Verification items for this drawing (mm, ordinates from the low corner). A direction names the side the tool comes from. Round coordinates to 2 decimals unless told otherwise and drop trailing zeros. Write each loop counter-clockwise with the first axis right and the second up, starting at its lowest first coordinate (ties: lowest second). Pieces come first, ordered by that corner, then holes. Notation, with made-up numbers: M 33,62 L 56,62 A18 ccw 56,85 Z; hole C 80,-14 d7. An arc over 180 degrees is marked long. Write each question's results on one line, items separated by ' | '.
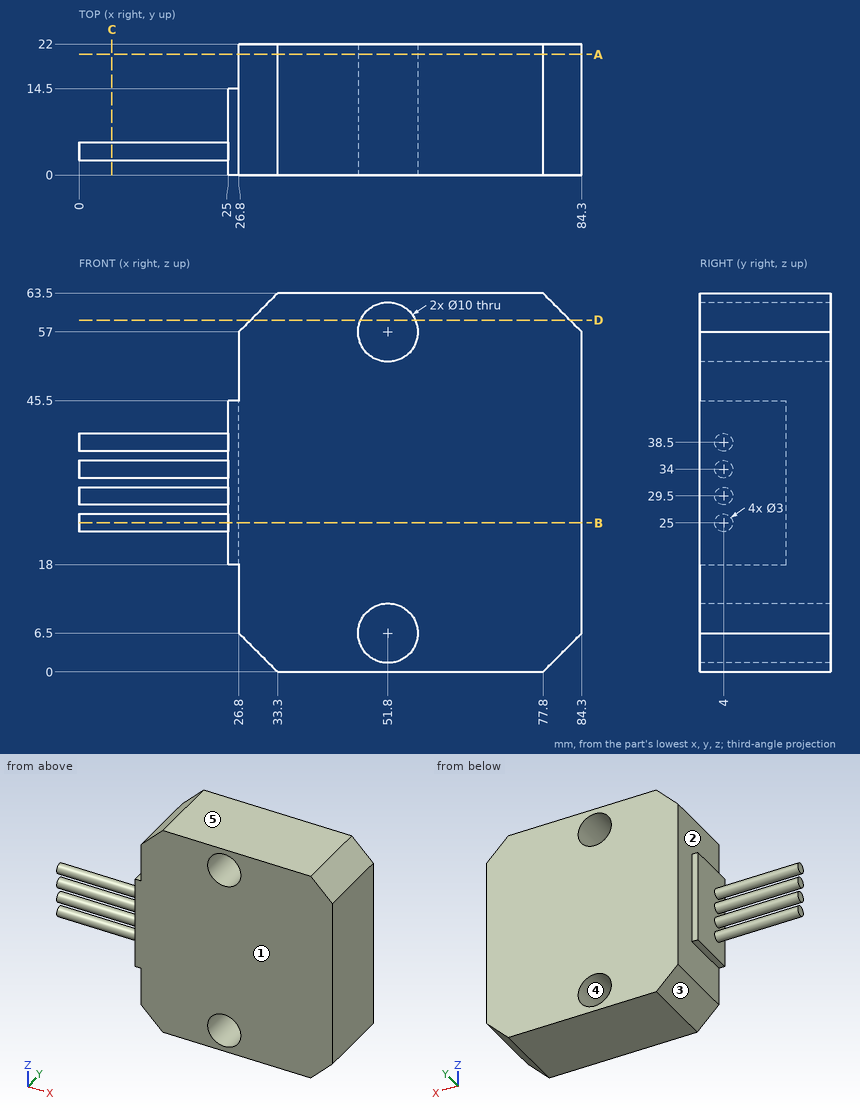
1) Material ranges on line 1 (X direction, y = 16.5, z = 6.5); line 2 (Z direction, x = 55, y = 16.75); line 3 (Z direction, x = 53, y = 4), recorded low to high. Write a range as [from, to].
Calculated:
line 1: x = [26.8, 46.8], [56.8, 84.3] | line 2: z = [0, 2.66], [10.34, 53.16], [60.84, 63.5] | line 3: z = [0, 1.65], [11.35, 52.15], [61.85, 63.5]
2) Access from +Z, -Z, +X, -X, +Y, -Y to the whole of each face (thin tool, end or side, straight path). Record for the marked faces 1 and 2.
Calculated:
face 1: +Z, -Z, +X, -X, -Y | face 2: -X, +Y
3) Sectioned sample at D-D, the plane z = 59. Record the cut outline in (x, y), and give its area (3 significant figures).
Calculated:
outline: M 28.8,0 L 47.22,0 L 47.22,22 L 28.8,22 Z; M 56.38,0 L 82.3,0 L 82.3,22 L 56.38,22 Z | area: 975 mm²
4) Sectioned sample at B-B, the plane z = 25. Record the cut outline in (x, y).
Calculated:
outline: M 0,2.5 L 25,2.5 L 25,0 L 84.3,0 L 84.3,22 L 26.8,22 L 26.8,14.5 L 25,14.5 L 25,5.5 L 0,5.5 Z
5) Draft check along X on the marked faces 3, 4 and 5. Enter one of: pulls with the +X half, pulls with the -X half, needs draft (parallel to the pull), parting line crosses it, or undercut.
Calculated:
face 3: pulls with the -X half | face 4: undercut | face 5: needs draft
6) Sectioned sample at C-C, the plane x = 5.5. Record the cut outline in (y, z).
Calculated:
outline: C 4,25 d3; C 4,29.5 d3; C 4,34 d3; C 4,38.5 d3
7) Depth check by flat-ended pin: P1, Ø6.5, axis at y = 10, z = 36.5, coming from the -X side; P2, Ø0.9, axis at x = 25.5, z = 28, coming from the +Y side; P3, Ø13, axis at x = 51.8, z = 6.5, coming from the +Y side; P4, Ø1, axis at y = 17.5, z = 14, coming from the -X side. Enter the tip coordinate at first touch or a pass-through.
Calculated:
P1: stops at x = 25 | P2: stops at y = 14.5 | P3: stops at y = 22 | P4: stops at x = 26.8
8) Sectioned sample at A-A, the plane y = 20.25. Record the cut outline in (x, z).
Calculated:
outline: M 26.8,6.5 L 33.3,0 L 77.8,0 L 84.3,6.5 L 84.3,57 L 77.8,63.5 L 33.3,63.5 L 26.8,57 Z; hole C 51.8,6.5 d10; hole C 51.8,57 d10
